Solid Edge part; units mm, degrees
sketch "Sketch1" plane through (0, 0, 0) normal (1, 0, 0) x (0, 1, 0)
  line L0 (7.5, 22) -> (7.5, 9)
  line L1 (7.5, 9) -> (20, 0)
  line L2 (20, 0) -> (0, 0)
  line L3 (0, 0) -> (0, 22)
  line L4 (0, 22) -> (0, 60)
  line L5 (0, 60) -> (7.5, 60)
  line L6 (7.5, 60) -> (7.5, 44)
  line L7 (7.5, 44) -> (6.5, 44)
  line L8 (6.5, 44) -> (6.5, 22)
  line L9 (7.5, 22) -> (6.5, 22)
  dimension "D1" = 20
  dimension "D2" = 7.5
revolve "RevolvedProtrusion1" add sketch "Sketch1" angle 360 about axis through (0, 0, 0) along (0, 0, 1)
The model under review builds one solid part; all positions refer to its coordinate system, in mm. A direction names the side the tool comes from. Round coordinates to 2 decimals unless told otherwise and drop trailing zeros. Loops run counter-clockwise (first coordinate to the right, second up) from the corner with the lowest first, then second, coordinate; pieces in that order, holes last. Notation, with made-up numbers: (-31.5, 67.25) - (-20.5, 67.25) arc R32 cw to (-20.5, 103.25) - close; hole circle Ø9 at (5.25, 14.25). An arc over 180 degrees is marked (long way). Use CSV: the item, a comma, the result in double quotes.
(1) Take a section at A-A, the plane y = 0. Give the boundary of the cut face in (x, z).
Working result:
outline,"(-20, 0) - (20, 0) - (7.5, 9) - (7.5, 22) - (6.5, 22) - (6.5, 44) - (7.5, 44) - (7.5, 60) - (-7.5, 60) - (-7.5, 44) - (-6.5, 44) - (-6.5, 22) - (-7.5, 22) - (-7.5, 9) - close"
(2) For line 1 (X direction, y = 0, z = 24.5); line 2 (Z direction, x = -1, y = -10); line 3 (Z direction, x = -12.5, y = -6), list the stretches that pass through material, from the lowest coordinate up.
Working result:
line 1,"x = -6.5 to 6.5"
line 2,"z = 0 to 7.16"
line 3,"z = 0 to 4.42"
(3) The part is to be moulded in two halves that separate along Z. For faces 4 (the flat face through (-3, -6, 22)), 5 (the cylindrical face through (0.33, -7.493, 51.888)), 6 (the flat face through (0, 0, 0)), say which applies: pulls with the +Z half, pulls with the -Z half, needs draft (parallel to the pull), parting line crosses it, or undercut.
Working result:
face 4,"undercut"
face 5,"needs draft"
face 6,"pulls with the -Z half"
(4) Take a section at C-C, the plane z = 56.5. Give the boundary of the cut face in (x, y), plus the area to 3 significant figures.
Working result:
outline,"circle Ø15 at (0, 0)"
area,"177 mm^2"
(5) Machinability: for faces 1 (the cylindrical face through (-3.955, -5.158, 32.846)), 2 (the cylindrical face through (0.33, -7.493, 15.409)), 3 (the flat face through (0, 0, 60)), which of the approach directions +Z, -Z, +X, -X, +Y, -Y give a long, thin tool a straight path to every point of the face, cutting with its end or side? Answer none if there is none.
Working result:
face 1,"none"
face 2,"+Z"
face 3,"+Z, +X, -X, +Y, -Y"
(6) Clearance check with flat-ended pins moving along their axes: P1, Ø5, axis at x = 6.5, y = -10.5, coming from the +Z side; P2, Ø8, axis at x = -1, z = 6.5, coming from the -Y side; P3, Ø1.5, axis at x = 13.5, y = -8, coming from the +Z side. State where each tip first meets the part, or that it passes through.
Working result:
P1,"stops at z = 7.31"
P2,"stops at y = -16.5"
P3,"stops at z = 3.64"
